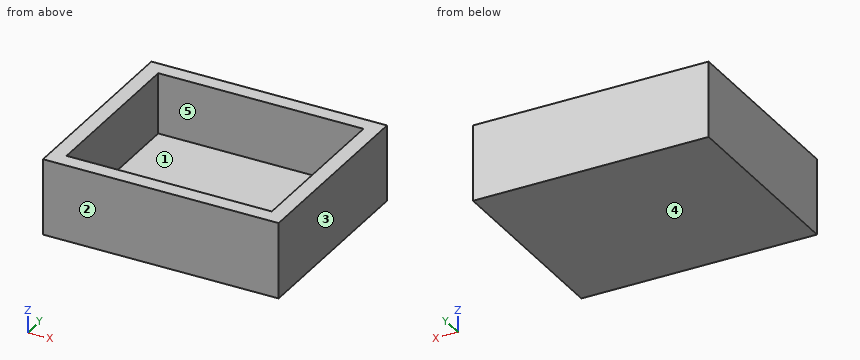
Autodesk Fusion 360 part; units mm, degrees
sketch "Sketch1" plane through (0, 0, 0) normal (0, 0, 1) x (1, 0, 0)
  line L0 (0, 0) -> (31, 0)
  line L1 (31, 0) -> (31, 26)
  line L2 (31, 26) -> (0, 26)
  line L3 (0, 26) -> (0, 0)
  dimension "d1" = 31
  dimension "d2" = 26
extrude "Extrude1" add sketch "Sketch1" along normal blind 10
shell "Shell1" thickness 2 removed faces 1 at (10.3333, 17.3333, 10)
extrude "Extrude2" cut 1 faces at (0, 17.3333, 3.3333) along direction (-1, 0, 0) blind 10
extrude "Extrude3" cut 1 faces at (31, 8.6667, 3.3333) along direction (1, 0, 0) blind 20
Build history of the part. All positions in model axes, mm. Face numbers are marked on the shaded views. A direction names the side the tool comes from. Coordinates: 2 decimals unless noted, no trailing zeros. Write each loop counter-clockwise with the first axis right and the second up, starting at its lowest first coordinate (ties: lowest second). Pieces come first, ordered by that corner, then holes.
1. Drill centre lines: probe 1 along Y at (x, z) = (13.5, 7.5); probe 2 along X at (y, z) = (12.75, 3.25); probe 3 along Z at (x, y) = (8, 19). Where is each one in solid material? Low to high.
Answer block:
probe 1: y = 0 to 2, 24 to 26
probe 2: x = 0 to 2, 29 to 31
probe 3: z = 0 to 2
2. Band-saw the part on C-C, the plane x = 20.5. Give the cut face in (y, z).
Answer block:
outline: (0, 0) - (26, 0) - (26, 10) - (24, 10) - (24, 2) - (2, 2) - (2, 10) - (0, 10) - close
3. Drop a flat-ended pin along its axis: pin 1 (6.5 mm diameter, centred on x = 18, y = 12, fed in from +Z). Give the stop position or say it passes through.
Answer block:
pin 1: stops at z = 2
4. Band-saw the part on B-B, the plane y = 4.5. Give the cut face in (x, z).
Answer block:
outline: (0, 0) - (31, 0) - (31, 10) - (29, 10) - (29, 2) - (2, 2) - (2, 10) - (0, 10) - close
5. Band-saw the part on A-A, the plane z = 7.5. Give the cut face in (x, y).
Answer block:
outline: (0, 0) - (31, 0) - (31, 26) - (0, 26) - close; hole (2, 2) - (29, 2) - (29, 24) - (2, 24) - close
6. Pull direction X, two halves, no side cores. Call the marked faces 3, 4 and 5: released by +X, released by -X, zero draft, split by the parting line, or undercut.
Answer block:
face 3: released by +X
face 4: zero draft
face 5: undercut
7. 3-axis set-ups, long thin cutter, end or side, ignore diameter. For the marked faces 1 and 2: which of +Z, -Z, +X, -X, +Y, -Y reach the whole face in a straight line?
Answer block:
face 1: +Z
face 2: +Z, -Z, +X, -X, -Y
